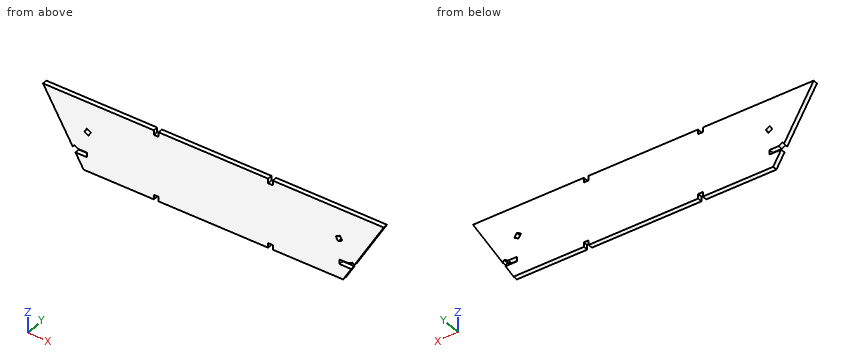
from build123d import *

# Parameters (mm, degrees)
BOSS_EXTRUDE1_DEPTH = 12.7
SKETCH2_OUTSIDE_W   = 2337.202
SKETCH2_OUTSIDE_H   = 2089.8
CUT_EXTRUDE1_DEPTH  = 12.7
SKETCH3_W           = 12.7
SKETCH3_H           = 12.7
CUT_EXTRUDE2_DEPTH  = 12.7
CUT_EXTRUDE3_DEPTH  = 12.7


with BuildPart() as part:
    # Sketch1 → Boss-Extrude1 (new body)
    with BuildSketch(Plane(origin=(0, 609.6, 0), x_dir=(1, 0, 0), z_dir=(0, 1, 0))):
        Polygon((923.311665212, 0), (461.655832606, 799.611357684), (-461.655832606, 799.611357684), (-923.311665212, 0), (-461.655832606, -799.611357684), (461.655832606, -799.611357684), align=None)
        Polygon((-351.670606325, 609.111357684), (-703.34121265, 0), (-351.670606325, -609.111357684), (351.670606325, -609.111357684), (703.34121265, 0), (351.670606325, 609.111357684), align=None, mode=Mode.SUBTRACT)
    extrude(amount=-BOSS_EXTRUDE1_DEPTH)

    # Sketch2 outside → Cut-Extrude1 (cut)
    with BuildSketch(Plane(origin=(0, 609.6, 0), x_dir=(1, 0, 0), z_dir=(0, 1, 0))):
        Rectangle(SKETCH2_OUTSIDE_W, SKETCH2_OUTSIDE_H)
        Polygon((-351.670606325, -609.111357684), (-461.655832606, -799.611357684), (461.655832606, -799.611357684), (351.670606325, -609.111357684), align=None, mode=Mode.SUBTRACT)
    extrude(amount=-CUT_EXTRUDE1_DEPTH, mode=Mode.SUBTRACT)

    # Sketch3 → Cut-Extrude2 (cut)
    with BuildSketch(Plane(origin=(0, 609.6, 0), x_dir=(1, 0, 0), z_dir=(0, 1, 0))):
        with Locations((-154.820606325, -615.461357684)):
            Rectangle(SKETCH3_W, SKETCH3_H)
        Polygon((-342.9, -725.902493452), (-331.901477372, -719.552493452), (-338.251477372, -708.553970824), (-349.25, -714.903970824), align=None)
        with Locations((-154.820606325, -793.261357684)):
            Rectangle(SKETCH3_W, SKETCH3_H)
        Polygon((-373.667651581, -647.211357684), (-381, -659.911357684), (-377.333825791, -666.261357684), (-366.335303163, -659.911357684), align=None)
        Polygon((381, -659.911357684), (373.667651581, -647.211357684), (366.335303163, -659.911357684), (377.333825791, -666.261357684), align=None)
        Polygon((338.251477372, -708.553970824), (331.901477372, -719.552493452), (342.9, -725.902493452), (349.25, -714.903970824), align=None)
        with Locations((154.820606325, -615.461357684)):
            Rectangle(SKETCH3_W, SKETCH3_H)
        with Locations((154.820606325, -793.261357684)):
            Rectangle(SKETCH3_W, SKETCH3_H)
    extrude(amount=-CUT_EXTRUDE2_DEPTH, mode=Mode.SUBTRACT)

    # Sketch4 → Cut-Extrude3 (cut)
    with BuildSketch(Plane(origin=(0, 609.6, 0), x_dir=(1, 0, 0), z_dir=(0, 1, 0))):
        Polygon((366.335303163, -659.911357684), (373.667651581, -647.211357684), (341.917651581, -647.211357684), (341.917651581, -659.911357684), align=None)
        Polygon((-373.667651581, -647.211357684), (-341.917651581, -647.211357684), (-341.917651581, -659.911357684), (-366.335303163, -659.911357684), align=None)
    extrude(amount=-CUT_EXTRUDE3_DEPTH, mode=Mode.SUBTRACT)


solid = part.part
Verification items for the finished model (mm, model axes). Round coordinates to 2 decimals unless told otherwise and drop trailing zeros. Order: outer loops, then holes, each group sorted by start corner. A loop starts at its lowest first (then second) coordinate and runs counter-clockwise, first axis right, second up.
1. Go/stop test with flat-tipped pins: P1, Ø6, axis at y = 602.5, z = 693.5, coming from the +X side; P2, Ø6.5, axis at y = 600.5, z = 656.5, coming from the +X side; P3, Ø4, axis at y = 600.5, z = 749, coming from the +X side. Record where each tip stops, or that it passes through.
Final values:
P1: stops at x = 402.12
P2: stops at x = 341.92
P3: stops at x = 433.59
2. Section check B-B on z = 680. Record the cut outline in (x, y).
Final values:
outline: (-392.6, 596.9) - (392.6, 596.9) - (392.6, 609.6) - (-392.6, 609.6) - close
3. Section check A-A on y = 606.5. State how many separate pieces and enclosed holes the cut face has, then the cut area to 3 significant figures.
Final values:
separate pieces: 1
enclosed holes: 2
area: 153,000 mm2
4. Section check C-C on z = 630.5. Record the cut outline in (x, y).
Final values:
outline: (-364.02, 596.9) - (364.02, 596.9) - (364.02, 609.6) - (-364.02, 609.6) - close
5. Thickness scan on L1, parallel to X at y = 607.75, z = 719; L2, parallel to X at y = 602.5, z = 652; L3, parallel to X at y = 598.75, z = 665. Record the ranges inside material, lowest first.
Final values:
L1: x = -415.11 to -346.89, -332.22 to 332.22, 346.89 to 415.11
L2: x = -341.92 to 341.92
L3: x = -383.94 to -378.06, -375.15 to 375.15, 378.06 to 383.94
